The model under review builds one solid part; all positions refer to its coordinate system, in mm. A direction names the side the tool comes from. Give positions to 0.01 mm unless a question says otherwise; leave off trailing zeros. Loops run counter-clockwise (first coordinate to the right, second up) from the corner with the lowest first, then second, coordinate; pieces in that order, holes last. Notation, with made-up numbers: (57, 41.5) - (102, 41.5) arc R15 cw to (102, 50.5) - close; hole circle Ø11 at (34, -30.75). An arc over 180 degrees is marked (long way). Answer as a JSON object with one key per item and string values.
from build123d import *

# Parameters (mm, degrees)
SKETCH_1_W                = 50.28
SKETCH_1_H                = 34.2
SKETCH_1_W_2              = 30.28
SKETCH_1_H_2              = 14.2
EXTRUDE_1_DEPTH           = 12.25
SKETCH_4_W                = 13
SKETCH_4_H                = 13.91
EXTRUDE_1_2_DEPTH         = 74.82
SKETCH_5_W                = 13.91
SKETCH_5_H                = 16.23
EXTRUDE_2_DEPTH           = 16
SKETCH_7_R                = 25.25
SKETCH_7_R_2              = 15.25
EXTRUDE_2_2_DEPTH         = 16.23
SKETCH_15_R               = 1.91
CUT_EXTRUDE_6_DEPTH       = 97.964478439
SKETCH_18_W               = 49.344544624
SKETCH_18_H               = 6.125
CUT_EXTRUDE_8_DEPTH       = 101.789238284
SKETCH_19_W               = 34.2
SKETCH_19_H               = 6.125
CUT_EXTRUDE_9_DEPTH       = 10
SKETCH_21_R               = 1.91
CUT_EXTRUDE_10_DEPTH      = 10
SKETCH_20_R               = 1.91
CUT_EXTRUDE_11_DEPTH      = 10
FILLET_START              = -7.1
FILLET_1_DEPTH            = 14.2
FILLET_2_DEPTH            = 14.2
SKETCH_29_W               = 13.91
SKETCH_29_H               = 74.82
EXTRUDE_5_DEPTH           = 10
SKETCH_30_W               = 10
SKETCH_30_H               = 58.59
CUT_EXTRUDE_13_DEPTH      = 97.964478439
SKETCH_32_W               = 34.2
SKETCH_32_H               = 5.745736365
EXTRUDE_6_DEPTH           = 10
CUT_EXTRUDE_16_DEPTH      = 50
CUT_EXTRUDE_16_DEPTH_BACK = 50
SKETCH_38_W               = 116.985630298
SKETCH_38_H               = 80.538350638
SKETCH_41_W               = 13.91
SKETCH_41_H               = 5.745736365
EXTRUDE_7_DEPTH           = 3
SKETCH_42_W               = 13
SKETCH_42_H               = 13.91
EXTRUDE_8_DEPTH           = 74.82
SKETCH_43_W               = 13.91
SKETCH_43_H               = 16.23
EXTRUDE_9_DEPTH           = 15.22
SKETCH_44_R               = 1.91
CUT_EXTRUDE_17_DEPTH      = 15.22
SKETCH_46_R               = 25.25
SKETCH_46_R_2             = 15.25
EXTRUDE_6_2_DEPTH         = 16.23
EXTRUDE_10_DEPTH          = 7.22
EXTRUDE_10_DEPTH_BACK     = 10
SKETCH_47_W               = 13.91
SKETCH_47_H               = 16.23
SKETCH_50_W               = 3.056753925
SKETCH_50_H               = 16.23
CUT_EXTRUDE_18_DEPTH      = 96.578211037
SKETCH_51_R               = 1.91
CUT_EXTRUDE_19_DEPTH      = 95.015226304


with BuildPart() as part:
    # 草圖1 → Extrude 1 (new body)
    with BuildSketch(Plane(origin=(0, 0, 0), x_dir=(1, 0, 0), z_dir=(0, 1, 0))):
        Rectangle(SKETCH_1_W, SKETCH_1_H)
        Rectangle(SKETCH_1_W_2, SKETCH_1_H_2, mode=Mode.SUBTRACT)
    extrude(amount=EXTRUDE_1_DEPTH)

    # 草圖4 → Extrude 1 2 (add)
    with BuildSketch(Plane.XZ):
        with Locations((18.64, 0)):
            Rectangle(SKETCH_4_W, SKETCH_4_H)
    extrude(amount=EXTRUDE_1_2_DEPTH)

    # 草圖5 → Extrude 2 (add)
    with BuildSketch(Plane.ZY.offset(-12.14)):
        with Locations((0, -66.705)):
            Rectangle(SKETCH_5_W, SKETCH_5_H)
    extrude(amount=EXTRUDE_2_DEPTH)

    # 草圖7 → Extrude 2 2 (add)
    with BuildSketch(Plane(origin=(3.626674765, -74.82, 0), x_dir=(1, 0, 0), z_dir=(0, -1, 0))):
        with Locations((-30.978154344, 0)):
            Circle(SKETCH_7_R)
        with Locations((-30.978154344, 0)):
            Circle(SKETCH_7_R_2, mode=Mode.SUBTRACT)
    extrude(amount=-EXTRUDE_2_2_DEPTH)

    # 草圖15 → 除料-伸長6 (cut, through all)
    with BuildSketch(Plane(origin=(0, 0, -6.955), x_dir=(-1, 0, 0), z_dir=(0, 0, -1))):
        with Locations((-4.530883248, -66.705)):
            Circle(SKETCH_15_R)
    extrude(amount=-CUT_EXTRUDE_6_DEPTH, mode=Mode.SUBTRACT)

    # 草圖18 → 除料-伸長8 (cut, through all)
    with BuildSketch(Plane(origin=(0, 0, -17.1), x_dir=(-1, 0, 0), z_dir=(0, 0, -1))):
        with Locations((0.467727688, 9.1875)):
            Rectangle(SKETCH_18_W, SKETCH_18_H)
    extrude(amount=-CUT_EXTRUDE_8_DEPTH, mode=Mode.SUBTRACT)

    # 草圖19 → 除料-伸長9 (cut)
    with BuildSketch(Plane.ZY.offset(-24.204544624)):
        with Locations((0, 9.1875)):
            Rectangle(SKETCH_19_W, SKETCH_19_H)
    extrude(amount=-CUT_EXTRUDE_9_DEPTH, mode=Mode.SUBTRACT)

    # 草圖21 → 除料-伸長10 (cut)
    with BuildSketch(Plane(origin=(0, 6.125, 0), x_dir=(1, 0, 0), z_dir=(0, 1, 0))):
        with Locations(Location((17.69, 0, 0), (0, 0, 270))):
            Circle(SKETCH_21_R)
    extrude(amount=-CUT_EXTRUDE_10_DEPTH, mode=Mode.SUBTRACT)

    # 草圖20 → 除料-伸長11 (cut)
    with BuildSketch(Plane(origin=(0, 6.125, 0), x_dir=(1, 0, 0), z_dir=(0, 1, 0))):
        with Locations(Location((-17.395, 0, 0), (0, 0, 270))):
            Circle(SKETCH_20_R)
    extrude(amount=-CUT_EXTRUDE_11_DEPTH, mode=Mode.SUBTRACT)

    # 圓角1: read off the stored shape, not the designer's step
    # 圓角1 outline → 圓角1 (cut)
    with BuildSketch(Plane.XY.offset(FILLET_START)):
        with BuildLine():
            add(Edge.make_bspline(
                [(-15.14, 0), (-21.974170252, 5.199829476), (-25.14, 5.745736365)],
                knots=[0, 0, 0, 0.664102345, 0.664102345, 0.664102345], degree=2, weights=[1, 2.223777218, 1.822127795]))
            Line((-15.14, 0), (-15.14, 6.125))
            Line((-15.14, 6.125), (-25.14, 6.125))
            Line((-25.14, 6.125), (-25.14, 5.745736365))
        make_face()
    extrude(amount=FILLET_1_DEPTH, mode=Mode.SUBTRACT)

    # 圓角2: read off the stored shape, not the designer's step
    # 圓角2 outline → 圓角2 (cut)
    with BuildSketch(Plane.XY.offset(FILLET_START)):
        with BuildLine():
            Line((15.14, 6.125), (15.14, 0))
            add(Edge.make_bspline(
                [(15.14, 0), (21.974170252, 5.199829476), (25.14, 5.745736365)],
                knots=[0, 0, 0, 0.664102345, 0.664102345, 0.664102345], degree=2, weights=[1, 2.223777218, 1.822127795]))
            Line((25.14, 5.745736365), (25.14, 6.125))
            Line((25.14, 6.125), (15.14, 6.125))
        make_face()
    extrude(amount=FILLET_2_DEPTH, mode=Mode.SUBTRACT)

    # 草圖29 → 填料-伸長5 (add)
    with BuildSketch(Plane(origin=(25.14, 0, 0), x_dir=(0, 0, -1), z_dir=(1, 0, 0))):
        with Locations((0, -37.41)):
            Rectangle(SKETCH_29_W, SKETCH_29_H)
    extrude(amount=EXTRUDE_5_DEPTH)

    # 草圖30 → 除料-伸長13 (cut, through all)
    with BuildSketch(Plane.XY.offset(6.955)):
        with Locations((17.14, -29.295)):
            Rectangle(SKETCH_30_W, SKETCH_30_H)
    extrude(amount=-CUT_EXTRUDE_13_DEPTH, mode=Mode.SUBTRACT)

    # 草圖32 → Extrude 6 (add)
    with BuildSketch(Plane(origin=(25.14, 0, 0), x_dir=(0, 0, -1), z_dir=(1, 0, 0))):
        with Locations((0, 2.872868182)):
            Rectangle(SKETCH_32_W, SKETCH_32_H)
    extrude(amount=EXTRUDE_6_DEPTH)

    # 草圖38 → 除料-伸長16 (cut, two sides: drawn at the far end of the back side and taken through both)
    with BuildSketch(Plane(origin=(0, 0, -6.955), x_dir=(-1, 0, 0), z_dir=(0, 0, -1)).offset(-CUT_EXTRUDE_16_DEPTH_BACK)):
        with Locations((7.268869252, -40.269175319)):
            Rectangle(SKETCH_38_W, SKETCH_38_H)
    extrude(amount=CUT_EXTRUDE_16_DEPTH + CUT_EXTRUDE_16_DEPTH_BACK, mode=Mode.SUBTRACT)

    # 草圖41 → 填料-伸長7 (add)
    with BuildSketch(Plane(origin=(35.14, 0, 0), x_dir=(0, 0, -1), z_dir=(1, 0, 0))):
        with Locations((0, 2.872868182)):
            Rectangle(SKETCH_41_W, SKETCH_41_H)
    extrude(amount=EXTRUDE_7_DEPTH)

    # 草圖42 → 填料-伸長8 (add)
    with BuildSketch(Plane(origin=(0, 0, 0), x_dir=(-1, 0, 0), z_dir=(0, -1, 0))):
        with Locations((-31.64, 0)):
            Rectangle(SKETCH_42_W, SKETCH_42_H)
    extrude(amount=EXTRUDE_8_DEPTH)

    # 草圖43 → 填料-伸長9 (add)
    with BuildSketch(Plane.ZY.offset(-25.14)):
        with Locations((0, -66.705)):
            Rectangle(SKETCH_43_W, SKETCH_43_H)
    extrude(amount=EXTRUDE_9_DEPTH)

    # 草圖44 → 除料-伸長17 (cut)
    with BuildSketch(Plane(origin=(0, 0, -6.955), x_dir=(-1, 0, 0), z_dir=(0, 0, -1))):
        with Locations(Location((-17.524895264, -66.705, 0), (0, 0, 90))):
            Circle(SKETCH_44_R)
    extrude(amount=-CUT_EXTRUDE_17_DEPTH, mode=Mode.SUBTRACT)

    # 草圖46 → Extrude 6 2 (add)
    with BuildSketch(Plane(origin=(0, -58.59, 0), x_dir=(1, 0, 0), z_dir=(0, 1, 0))):
        with Locations((-14.35, 0)):
            Circle(SKETCH_46_R)
        with Locations((-14.35, 0)):
            Circle(SKETCH_46_R_2, mode=Mode.SUBTRACT)
    extrude(amount=-EXTRUDE_6_2_DEPTH)

    # 草圖47 → 填料-伸長10 (add, two sides: drawn at the far end of the back side and taken through both)
    with BuildSketch(Plane(origin=(-40, 0, 0), x_dir=(0, 0, -1), z_dir=(1, 0, 0)).offset(-EXTRUDE_10_DEPTH_BACK)):
        with Locations((0, -66.705)):
            Rectangle(SKETCH_47_W, SKETCH_47_H)
    extrude(amount=EXTRUDE_10_DEPTH + EXTRUDE_10_DEPTH_BACK)

    # 草圖50 → 除料-伸長18 (cut, through all)
    with BuildSketch(Plane(origin=(0, 0, -6.955), x_dir=(-1, 0, 0), z_dir=(0, 0, -1))):
        with Locations((48.471623038, -66.705)):
            Rectangle(SKETCH_50_W, SKETCH_50_H)
    extrude(amount=-CUT_EXTRUDE_18_DEPTH, mode=Mode.SUBTRACT)

    # 草圖51 → 除料-伸長19 (cut, through all)
    with BuildSketch(Plane(origin=(0, 0, -6.955), x_dir=(-1, 0, 0), z_dir=(0, 0, -1))):
        with Locations((42.786508152, -66.705)):
            Circle(SKETCH_51_R)
    extrude(amount=-CUT_EXTRUDE_19_DEPTH, mode=Mode.SUBTRACT)


solid = part.part
Q1. Consider section B-B, the plane z = 14. State the section outline as (x, y) points (3 decimals), plus the area to 3 significant figures.
Results:
{"outline": "(-35.363, -74.82) - (-20.397, -74.82) - (-20.397, -58.59) - (-35.363, -58.59) - close; (-25.14, 0) - (35.14, 0) - (35.14, 5.746) - (25.14, 5.746) - (25.14, 6.125) - (-25.14, 6.125) - close; (-8.303, -74.82) - (6.663, -74.82) - (6.663, -58.59) - (-8.303, -58.59) - close", "area": "851 mm^2"}
Q2. Consider section D-D, the plane y = -40. State the section outline as (x, z) points (3 decimals).
Results:
{"outline": "(25.14, -6.955) - (38.14, -6.955) - (38.14, 6.955) - (25.14, 6.955) - close"}
Q3. Consider section A-A, the plane x = 12. State the section outline as (y, z) points (3 decimals), plus the area to 3 significant figures.
Results:
{"outline": "(-74.82, -6.955) - (-58.59, -6.955) - (-58.59, 6.955) - (-74.82, 6.955) - close; (0, -17.1) - (6.125, -17.1) - (6.125, -7.1) - (0, -7.1) - close; (0, 7.1) - (6.125, 7.1) - (6.125, 17.1) - (0, 17.1) - close", "area": "348 mm^2"}
Q4. Clearance check with flat-ended pins moving along their axes: pin 1 Ø6.5 at (x, z) = (30.5, -7) entering from +Y; pin 2 Ø5 at (x, z) = (-36, -14.5) entering from +Y; pin 3 Ø6.5 at (x, y) = (1, 2) entering from +Z. State where each tip first meets the part, or that it passes through.
Results:
{"pin 1": "stops at y = 5.75", "pin 2": "stops at y = -58.59", "pin 3": "stops at z = 17.1"}
Q5. The part is to be moulded in two halves that separate along Y. For faces 5 (the face through (4, -74.82, 0)), 6 (the face through (-43, -69, -6.955)), 7 (the face through (0, 6.125, 12)), 8 (the face through (25.14, -29, 0)), say which applies: +Y half, -Y half, draft (parallel to the pull), parting line (faces both ways), or undercut.
Results:
{"face 5": "-Y half", "face 6": "draft", "face 7": "+Y half", "face 8": "undercut"}
Q6. For faces 1 (the face through (-13.893, -66.591, -25.246)), 2 (the face through (-0.263, -66.591, 5.841)), 3 (the face through (-43, -69, 6.955)), 4 (the face through (-25.14, 3, 0)), list the 3-axis set-ups (+Z, -Z, +X, -X, +Y, -Y) from which the entire face can be reached by the end or side of a thin tool; tool diameter is ignored.
Results:
{"face 1": "-Z, -Y", "face 2": "-Y", "face 3": "+Z, -X, +Y, -Y", "face 4": "+Z, -Z, -X, +Y"}
Q7. To check wall thickness, follow probe 1 along X at (y, z) = (1, 0) (3 decimals); probe 2 along Z at (x, y) = (17.69, 1.3); probe 3 along Z at (x, y) = (-14, -67). State the ranges of each line that lie inside material, in increasing order. Write a range as [from, to].
Results:
{"probe 1": "x = [-25.14, -19.305], [19.6, 38.14]", "probe 2": "z = [-17.1, -1.91], [1.91, 17.1]", "probe 3": "z = [-25.25, -15.25], [15.25, 25.25]"}
Q8. Consider section C-C, the plane x = -8.5. State the section outline as (y, z) points (3 decimals), plus the area to 3 significant figures.
Results:
{"outline": "(-74.82, -24.563) - (-58.59, -24.563) - (-58.59, -14.083) - (-74.82, -14.083) - close; (-74.82, 14.083) - (-58.59, 14.083) - (-58.59, 24.563) - (-74.82, 24.563) - close; (0, -17.1) - (6.125, -17.1) - (6.125, -7.1) - (0, -7.1) - close; (0, 7.1) - (6.125, 7.1) - (6.125, 17.1) - (0, 17.1) - close", "area": "463 mm^2"}
